Could you check a few things on this model? Use its own coordinates, in mm. Face numbers are marked on the shaded views. A direction names the side the tool comes from. Round coordinates to 2 decimals unless told otherwise and drop trailing zeros. Write each loop counter-clockwise with the first axis right and the second up, starting at its lowest first coordinate (ties: lowest second). Pieces come first, ordered by that corner, then holes. Notation, with made-up numbers: (-10.5, -35.75) -> (-5.5, -35.75) arc R27 ccw to (-5.5, -3.75) -> close; hole circle Ø7 at (73, 41). An arc over 180 degrees is marked (long way). Answer in a Markdown table with one row per item.
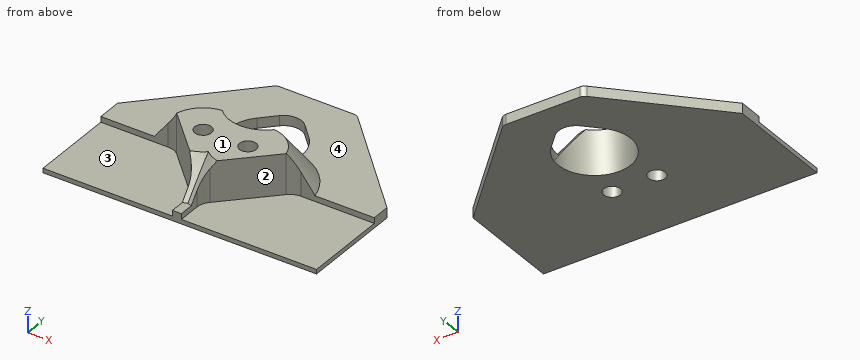
from build123d import *

# Parameters (mm, degrees)
CYLINDER_R       = 1.5
CYLINDER_DEPTH   = 8
ARRAY001_COUNT   = 4
ARRAY004_COUNT   = 4
EXTRUDE003_DEPTH = 1.8
EXTRUDE002_DEPTH = 0.8
ARRAY006_COUNT   = 4
EXTRUDE_DEPTH    = 1
ARRAY002_COUNT   = 4
EXTRUDE006_DEPTH = 1.8
EXTRUDE004_DEPTH = 10
EXTRUDE001_DEPTH = 8
ARRAY005_COUNT   = 4
ARRAY_COUNT      = 4
ARRAY003_COUNT   = 4
SKETCH003_W      = 48.922418
SKETCH003_H      = 39.225639
EXTRUDE005_DEPTH = 10


with BuildPart() as holes:
    # Cylinder → Cylinder (new body)
    with BuildSketch(Plane(origin=(4, 4, 0), x_dir=(1, 0, 0), z_dir=(0, 0, 1))):
        Circle(CYLINDER_R)
    extrude(amount=CYLINDER_DEPTH)

    # Array001: holes ×4 about axis
    array001_axis = Axis((50, 50, 0), (0, 0, 1))


with BuildPart() as holes_1:
    add(holes.part)
    for i in range(1, ARRAY001_COUNT):
        add(holes.part.rotate(array001_axis, i * 360 / ARRAY001_COUNT))

    # Array004: holes ×4 about axis
    array004_axis = Axis((0, 0, 0), (0, 0, 1))


with BuildPart() as holes_2:
    add(holes_1.part)
    for i in range(1, ARRAY004_COUNT):
        add(holes_1.part.rotate(array004_axis, i * 360 / ARRAY004_COUNT))


with BuildPart() as top_hook:
    # Sketch002 → Extrude003 (new body)
    with BuildSketch(Plane.XY):
        with BuildLine():
            Line((26.654903, 100), (7.555178, 119.595928))
            ThreePointArc((7.555178, 119.595928), (7.116991, 119.89485), (6.597081, 120))
            Line((6.597081, 120), (0, 120))
            Line((-6.597081, 120), (0, 120))
            ThreePointArc((-6.597081, 120), (-7.116991, 119.89485), (-7.555178, 119.595928))
            Line((-7.555178, 119.595928), (-26.654903, 100))
            Line((-26.654903, 100), (0, 100))
            Line((0, 100), (26.654903, 100))
        make_face()
        with BuildLine():
            ThreePointArc((-4.654749, 111.036883), (0, 100), (4.654749, 111.036883))
            Line((2.294641, 113.458306), (4.654749, 111.036883))
            ThreePointArc((2.294641, 113.458306), (0, 114.426059), (-2.294641, 113.458306))
            Line((-4.654749, 111.036883), (-2.294641, 113.458306))
        make_face(mode=Mode.SUBTRACT)
    extrude(amount=EXTRUDE003_DEPTH)


with BuildPart() as extrude002:
    # Sketch001 → Extrude002 (new body)
    with BuildSketch(Plane.XY):
        with BuildLine():
            Line((0, 100), (96, 100))
            ThreePointArc((98.828427, 98.828427), (97.530734, 99.695518), (96, 100))
            Line((96, 96), (98.828427, 98.828427))
            Line((4, 4), (96, 96))
            Line((0, 0), (4, 4))
            Line((0, 0), (0, 100))
        make_face()
    extrude(amount=EXTRUDE002_DEPTH)


with BuildPart() as bottom_plate:
    # Part__Mirroring002: instance of Extrude002
    add(extrude002.part.mirror(Plane(origin=(0, 0, 0), x_dir=(1, 0, 0), z_dir=(0, 1, 0))))

    # Fusion003: union Extrude002
    add(extrude002.part)

    # Array006: bottom_plate ×4 about axis
    array006_axis = Axis((0, 0, 0), (0, 0, 1))


with BuildPart() as bottom_plate_1:
    add(bottom_plate.part)
    for i in range(1, ARRAY006_COUNT):
        add(bottom_plate.part.rotate(array006_axis, i * 360 / ARRAY006_COUNT))


with BuildPart() as extrude_body:
    # Sketch → Extrude (new body)
    with BuildSketch(Plane.XY):
        with BuildLine():
            Line((0, 100), (96, 100))
            ThreePointArc((98.828427, 98.828427), (97.530734, 99.695518), (96, 100))
            Line((96, 96), (98.828427, 98.828427))
            Line((4, 4), (96, 96))
            Line((0, 0), (4, 4))
            Line((0, 0), (0, 100))
        make_face()
        with BuildLine():
            Line((0.8, 10.565655), (0.8, 87.314719))
            ThreePointArc((1.67868, 89.436039), (1.028361, 88.462769), (0.8, 87.314719))
            Line((9.763961, 97.52132), (1.67868, 89.436039))
            ThreePointArc((11.885281, 98.4), (10.737231, 98.171639), (9.763961, 97.52132))
            Line((11.885281, 98.4), (90.032525, 98.4))
            ThreePointArc((92.151931, 93.283302), (92.801662, 96.549722), (90.032525, 98.4))
            Line((6.905361, 8.036732), (92.151931, 93.283302))
            ThreePointArc((0.8, 10.565655), (3.007794, 7.261458), (6.905361, 8.036732))
        make_face(mode=Mode.SUBTRACT)
    extrude(amount=EXTRUDE_DEPTH)


with BuildPart() as extrude_body_1:
    # Extrude placement: moved
    add(extrude_body.part.moved(Location((0, 0, 0.8))))


with BuildPart() as fusion002:
    # Part__Mirroring: instance of Extrude body
    add(extrude_body_1.part.mirror(Plane(origin=(0, 0, 0), x_dir=(1, 0, 0), z_dir=(0, 1, 0))))

    # Fusion: union Extrude body
    add(extrude_body_1.part)

    # Array002: Fusion002 ×4 about axis
    array002_axis = Axis((0, 0, 0), (0, 0, 1))


with BuildPart() as fusion002_1:
    add(fusion002.part)
    for i in range(1, ARRAY002_COUNT):
        add(fusion002.part.rotate(array002_axis, i * 360 / ARRAY002_COUNT))

    # Fusion002: union bottom_plate
    add(bottom_plate_1.part)


with BuildPart() as extrude006:
    # Sketch004 → Extrude006 (new body)
    with BuildSketch(Plane.XY):
        with BuildLine():
            Line((-65.833333, 100), (-50, 100))
            Line((-50, 100), (-50, 120))
            Line((-71.666667, 120), (-50, 120))
            ThreePointArc((-71.666667, 120), (-75, 116.666667), (-71.666667, 113.333333))
            Line((-65.833333, 113.333333), (-71.666667, 113.333333))
            ThreePointArc((-62.5, 110), (-63.476311, 112.357023), (-65.833333, 113.333333))
            Line((-62.5, 103.333333), (-62.5, 110))
            ThreePointArc((-65.833333, 100), (-63.476311, 100.976311), (-62.5, 103.333333))
        make_face()
    extrude(amount=EXTRUDE006_DEPTH)


with BuildPart() as part_mirroring003:
    # Part__Mirroring003: instance of Extrude006
    add(extrude006.part.mirror(Plane(origin=(-50, 0, 0), x_dir=(0, -1, 0), z_dir=(1, 0, 0))))


with BuildPart() as cable_hook:
    # Fusion006 base: copy of Extrude006
    add(extrude006.part)

    # Fusion006: union Part__Mirroring003
    add(part_mirroring003.part)


with BuildPart() as hook_zone:
    # Sketch002 → Extrude004 (new body)
    with BuildSketch(Plane.XY):
        with BuildLine():
            Line((26.654903, 100), (7.555178, 119.595928))
            ThreePointArc((7.555178, 119.595928), (7.116991, 119.89485), (6.597081, 120))
            Line((6.597081, 120), (0, 120))
            Line((-6.597081, 120), (0, 120))
            ThreePointArc((-6.597081, 120), (-7.116991, 119.89485), (-7.555178, 119.595928))
            Line((-7.555178, 119.595928), (-26.654903, 100))
            Line((-26.654903, 100), (0, 100))
            Line((0, 100), (26.654903, 100))
        make_face()
        with BuildLine():
            ThreePointArc((-4.654749, 111.036883), (0, 100), (4.654749, 111.036883))
            Line((2.294641, 113.458306), (4.654749, 111.036883))
            ThreePointArc((2.294641, 113.458306), (0, 114.426059), (-2.294641, 113.458306))
            Line((-4.654749, 111.036883), (-2.294641, 113.458306))
        make_face(mode=Mode.SUBTRACT)
    extrude(amount=EXTRUDE004_DEPTH)


with BuildPart() as extrude001:
    # Sketch → Extrude001 (new body)
    with BuildSketch(Plane.XY):
        with BuildLine():
            Line((0, 100), (96, 100))
            ThreePointArc((98.828427, 98.828427), (97.530734, 99.695518), (96, 100))
            Line((96, 96), (98.828427, 98.828427))
            Line((4, 4), (96, 96))
            Line((0, 0), (4, 4))
            Line((0, 0), (0, 100))
        make_face()
        with BuildLine():
            Line((0.8, 10.565655), (0.8, 87.314719))
            ThreePointArc((1.67868, 89.436039), (1.028361, 88.462769), (0.8, 87.314719))
            Line((9.763961, 97.52132), (1.67868, 89.436039))
            ThreePointArc((11.885281, 98.4), (10.737231, 98.171639), (9.763961, 97.52132))
            Line((11.885281, 98.4), (90.032525, 98.4))
            ThreePointArc((92.151931, 93.283302), (92.801662, 96.549722), (90.032525, 98.4))
            Line((6.905361, 8.036732), (92.151931, 93.283302))
            ThreePointArc((0.8, 10.565655), (3.007794, 7.261458), (6.905361, 8.036732))
        make_face(mode=Mode.SUBTRACT)
    extrude(amount=EXTRUDE001_DEPTH)


with BuildPart() as zone_to_cut:
    # Part__Mirroring001: instance of Extrude001
    add(extrude001.part.mirror(Plane(origin=(0, 0, 0), x_dir=(1, 0, 0), z_dir=(0, 1, 0))))

    # Fusion001: union Extrude001
    add(extrude001.part)

    # Array005: zone_to_cut ×4 about axis
    array005_axis = Axis((0, 0, 0), (0, 0, 1))


with BuildPart() as zone_to_cut_1:
    add(zone_to_cut.part)
    for i in range(1, ARRAY005_COUNT):
        add(zone_to_cut.part.rotate(array005_axis, i * 360 / ARRAY005_COUNT))

    # Fusion004: union hook_zone
    add(hook_zone.part)


with BuildPart() as cut:
    # Cone → Cone (revolve)
    with BuildSketch(Plane(origin=(4, 4, 0), x_dir=(1, 0, 0), z_dir=(0, -1, 0))):
        Polygon((0, 0), (12, 0), (6, 8), (0, 8), align=None)
    revolve(axis=Axis((4, 4, 0), (0, 0, 1)))

    # Array: Cut ×4 about axis
    array_axis = Axis((50, 50, 0), (0, 0, 1))


with BuildPart() as cut_1:
    add(cut.part)
    for i in range(1, ARRAY_COUNT):
        add(cut.part.rotate(array_axis, i * 360 / ARRAY_COUNT))

    # Array003: Cut ×4 about axis
    array003_axis = Axis((0, 0, 0), (0, 0, 1))


with BuildPart() as cut_2:
    add(cut_1.part)
    for i in range(1, ARRAY003_COUNT):
        add(cut_1.part.rotate(array003_axis, i * 360 / ARRAY003_COUNT))

    # Common001: intersect zone_to_cut
    add(zone_to_cut_1.part, mode=Mode.INTERSECT)

    # Fusion005: union top_hook, Fusion002, cable_hook
    add(top_hook.part)
    add(fusion002_1.part)
    add(cable_hook.part)

    # Cut: cut holes
    add(holes_2.part, mode=Mode.SUBTRACT)


with BuildPart() as test_print:
    # Sketch003 → Extrude005 (new body)
    with BuildSketch(Plane.XY):
        with Locations((0.518458, 102.847819)):
            Rectangle(SKETCH003_W, SKETCH003_H)
    extrude(amount=EXTRUDE005_DEPTH)

    # Common: intersect Cut
    add(cut_2.part, mode=Mode.INTERSECT)


solid = test_print.part
1) Imagine slicing it at B-B, the plane y = 96. Please give me the cut outline in (x, z).
Findings:
| item | result |
|---|---|
| outline | (-23.94, 0) -> (-5.5, 0) -> (-5.5, 8) -> (-8.24, 8) -> (-8.24, 0.8) -> (-23.94, 0.8) -> close; (-2.5, 0) -> (2.5, 0) -> (2.5, 8) -> (-2.5, 8) -> close; (5.5, 0) -> (24.98, 0) -> (24.98, 0.8) -> (8.24, 0.8) -> (8.24, 8) -> (5.5, 8) -> close |
2) Please list where these lines run through material, in increasing order: line 1 (X direction, y = 96, z = 4); line 2 (X direction, y = 97, z = 3.25); line 3 (Z direction, x = 8.5, y = 88).
Findings:
| item | result |
|---|---|
| line 1 | x = -8.24 to -5.5, -2.5 to 2.5, 5.5 to 8.24 |
| line 2 | x = -9.24 to -5.12, -2.88 to 2.88, 5.12 to 9.24 |
| line 3 | z = 0 to 0.8 |
3) For the marked faces 1, 2, 3 and 4, which set-ups out of +Z, -Z, +X, -X, +Y, -Y let a thin tool reach every point of the face, with its end or its side?
Findings:
| item | result |
|---|---|
| face 1 | +Z, +X, -X, +Y, -Y |
| face 2 | +Z, +X, -Y |
| face 3 | +Z, -X, -Y |
| face 4 | +Z, +Y |
4) For pin 1 (0.8 mm diameter, centred on x = 0.5, y = 85, fed in from +Z); pin 2 (1.4 mm diameter, centred on y = 86, z = 2, fed in from +X); pin 3 (3.5 mm diameter, centred on x = -17, z = 3, fed in from -Y); pin 4 (1.8 mm diameter, centred on x = 4, y = 96, fed in from +Z), each with a flat end and sliding along its axis, tell me the tip position at first contact or that it passes through.
Findings:
| item | result |
|---|---|
| pin 1 | stops at z = 1.8 |
| pin 2 | stops at x = 0.8 |
| pin 3 | stops at y = 98.4 |
| pin 4 | passes through |
5) Imagine slicing it at A-A, the plane x = -4. Please give me the cut outline in (y, z) (3 decimals).
Findings:
| item | result |
|---|---|
| outline | (83.235, 0) -> (94.5, 0) -> (94.5, 8) -> (91.757, 8) -> (91.757, 0.8) -> (83.235, 0.8) -> close; (97.5, 0) -> (101.377, 0) -> (101.377, 8) -> (97.5, 8) -> close; (111.709, 0) -> (120, 0) -> (120, 1.8) -> (111.709, 1.8) -> close |
6) Imagine slicing it at C-C, the plane x = 16. Please give me the cut outline in (y, z) (3 decimals).
Findings:
| item | result |
|---|---|
| outline | (83.235, 0) -> (110.932, 0) -> (110.932, 1.8) -> (98.4, 1.8) -> (98.4, 0.8) -> (83.235, 0.8) -> close |
